Part model, mm, in its own coordinate system. A direction names the side the tool comes from. Give positions to 0.01 mm unless a question says otherwise; leave off trailing zeros. Write each loop counter-clockwise with the first axis right and the second up, starting at its lowest first coordinate (ties: lowest second). Pieces come first, ordered by that corner, then holes. Notation, with made-up numbers: (18.25, 88) - (50.25, 88) arc R15 cw to (50.25, 92) - close; hole circle Ø1 at (60.25, -24). An arc over 180 degrees is marked (long way). Answer as a JSON object with one key per item and string values. Group by question number.
```python
from build123d import *

# Parameters (mm, degrees)
F0_W     = 19.05
F0_H     = 203.2
F0_W_2   = 203.2
F0_H_2   = 19.05
F1_DEPTH = 19.05


with BuildPart() as f1:
    # F0 (on Front) → F1 (new body)
    with BuildSketch(Plane.XZ):
        with Locations((-434.523107, 137.960202)):
            Rectangle(F0_W, F0_H)
        Polygon((-164.648107, 391.960202), (-424.998107, 391.960202), (-424.998107, 239.560202), (-424.998107, 36.360202), (-424.998107, -96.989798), (-164.648107, -96.989798), (38.551893, -96.989798), (298.901893, -96.989798), (298.901893, 36.360202), (298.901893, 239.560202), (298.901893, 391.960202), (38.551893, 391.960202), (38.551893, 372.910202), (-164.648107, 372.910202), align=None)
        with BuildLine():
            ThreePointArc((-304.348107, 201.460202), (-291.648107, 214.160202), (-278.948107, 201.460202))
            ThreePointArc((-278.948107, 201.460202), (-278.961817, 200.870249), (-279.002917, 200.28157))
            Line((-279.002917, 200.28157), (-278.948108, 74.465734))
            ThreePointArc((-278.948108, 74.465734), (-278.948107, 74.462968), (-278.948107, 74.460202))
            ThreePointArc((-278.948107, 74.460202), (-291.648107, 61.760202), (-304.348107, 74.460202))
            Line((-304.348107, 74.460202), (-304.348107, 201.460202))
        make_face(mode=Mode.SUBTRACT)
        with Locations((308.426893, 137.960202)):
            Rectangle(F0_W, F0_H)
        with Locations((-63.048107, -106.514798)):
            Rectangle(F0_W_2, F0_H_2)
    extrude(amount=F1_DEPTH)


solid = f1.part
```
1) Two-plate mould, pull along Z, no slides. Class faces 4 (the flat face through (-435, -9, 239.56)), 5 (the cylindrical face through (-291.927, -9.392, 214.157)), 6 (the flat face through (298.902, -9, 315)): +Z half, -Z half, draft (parallel to the pull), parting line (faces both ways), or undercut.
2) Saw through at D-D (x = -316). List the corners of the cut face in (y, z).
3) Drop flat-ended pins along their axis: P1, Ø8, axis at x = -41.5, y = -14.5, coming from the +Z side; P2, Ø9.5, axis at x = 130.5, y = -14, coming from the -Z side; P3, Ø5.5, axis at y = -6.5, z = -102, coming from the -X side. Give the stop position or say it passes through.
4) Saw through at B-B (z = 186.5). List the corners of the cut face in (x, y).
5) Saw through at C-C (z = 83.5). List the corners of the cut face in (x, y).
6) Drill centre lines: line 1 along Z through (x, y) = (-291, -10.75); line 2 along X through (y, z) = (-1.75, 171.5); line 3 along Z through (x, y) = (-178, -8). Where is each one in solid material? Low to high. Write a range as from..to.
7) Which spindle directions (+Z, -Z, +X, -X, +Y, -Y) get a long thin tool onto all of the face, cutting with end or side? Do faces 1 (the cylindrical face through (-291.369, -9.392, 61.763)), 2 (the flat face through (308, -9, 36.36)), 3 (the flat face through (-424.998, -9, -29)). Say none if no direction does.
Checks:
{
 "1": {"face 4": "+Z half", "face 5": "undercut", "face 6": "draft"},
 "2": {"outline": "(-19.05, -96.99) - (0, -96.99) - (0, 391.96) - (-19.05, 391.96) - close"},
 "3": {"P1": "z = 372.91", "P2": "z = -96.99", "P3": "x = -164.65"},
 "4": {"outline": "(-444.05, -19.05) - (-304.35, -19.05) - (-304.35, 0) - (-444.05, 0) - close; (-279, -19.05) - (317.95, -19.05) - (317.95, 0) - (-279, 0) - close"},
 "5": {"outline": "(-444.05, -19.05) - (-304.35, -19.05) - (-304.35, 0) - (-444.05, 0) - close; (-278.95, -19.05) - (317.95, -19.05) - (317.95, 0) - (-278.95, 0) - close"},
 "6": {"line 1": "-96.99..61.78, 214.14..391.96", "line 2": "-444.05..-304.35, -278.99..317.95", "line 3": "-96.99..391.96"},
 "7": {"face 1": "+Y, -Y", "face 2": "-Z, +X, +Y, -Y", "face 3": "-Z, -X, +Y, -Y"}
}
